Geometry check sheet. Reference: the model listing, model coordinates, mm. Face numbers are marked on the shaded views. A direction names the side the tool comes from. Round coordinates to 2 decimals unless told otherwise and drop trailing zeros. Order: outer loops, then holes, each group sorted by start corner. A loop starts at its lowest first (then second) coordinate and runs counter-clockwise, first axis right, second up.
(1) Cross-section at B-B on x = -2.5. Enter the section's corners in (y, z), and give its area (3 significant figures).
(2) Cross-section at C-C on x = 3.5. Enter the section's corners in (y, z), and give its area (4 significant figures).
(3) Gauge pin test, flat ends, axial feed: P1, Ø3, axis at x = -2.5, z = 4, coming from the -Y side; P2, Ø2, axis at x = -2.5, z = 4, coming from the -Y side. Record the tip position at first contact, or that the pin passes through.
(4) Cross-section at A-A on y = -4.25. Enter the section's corners in (x, z), and give its area (3 significant figures).
(5) Thickness scan on L1, parallel to X at y = -6, z = 4; L2, parallel to X at y = 4.25, z = 1.75; L3, parallel to Y at x = -2.75, z = 5. Record the ranges inside material, lowest first.
(6) Cross-section at D-D on z = 4.5. Enter the section's corners in (x, y).
(7) Draft check along X on the marked faces 1, 2 and 3. Enter one of: pulls with the +X half, pulls with the -X half, needs draft (parallel to the pull), parting line crosses it, or undercut.
(8) Set-up check for the marked faces 4 and 5: record each of +Z, -Z, +X, -X, +Y, -Y from which the full face is reachable in a straight line by a thin tool's end or side.
from build123d import *

# Parameters (mm, degrees)
SKETCH_1_W          = 12.7
SKETCH_1_H          = 15
EXTRUDE_1_DEPTH     = 8
SKETCH_2_R          = 0.75
CUT_EXTRUDE_1_DEPTH = 8
SKETCH_3_R          = 1.25
CUT_EXTRUDE_2_DEPTH = 5


with BuildPart() as part:
    # Эскиз1 → Бобышка-Вытянуть1 (new body)
    with BuildSketch(Plane.XY):
        Rectangle(SKETCH_1_W, SKETCH_1_H)
    extrude(amount=EXTRUDE_1_DEPTH)

    # Эскиз2 → Вырез-Вытянуть1 (cut)
    with BuildSketch(Plane.XY.offset(8)):
        with Locations((-2.3876, 3.786)):
            Circle(SKETCH_2_R)
        with Locations((2.3876, 3.79)):
            Circle(SKETCH_2_R)
    extrude(amount=-CUT_EXTRUDE_1_DEPTH, mode=Mode.SUBTRACT)

    # Эскиз3 → Вырез-Вытянуть2 (cut)
    with BuildSketch(Plane.XZ.offset(7.5)):
        with Locations(Location((-2.5, 4, 0), (0, 0, 270))):
            Circle(SKETCH_3_R)
        with Locations(Location((2.5, 4, 0), (0, 0, 270))):
            Circle(SKETCH_3_R)
    extrude(amount=-CUT_EXTRUDE_2_DEPTH, mode=Mode.SUBTRACT)


solid = part.part
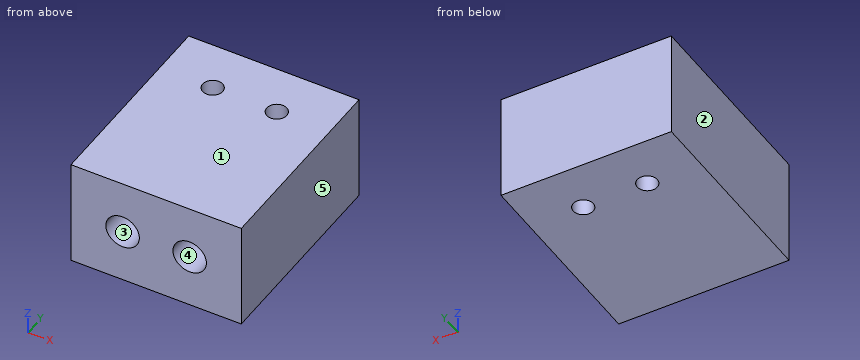
Found:
1. outline: (-7.5, 0) - (3.04, 0) - (3.04, 8) - (-7.5, 8) - (-7.5, 5.25) - (-2.5, 5.25) - (-2.5, 2.75) - (-7.5, 2.75) - close; (4.53, 0) - (7.5, 0) - (7.5, 8) - (4.53, 8) - close
1. area: 95.6 mm2
2. outline: (-7.5, 0) - (7.5, 0) - (7.5, 8) - (-7.5, 8) - (-7.5, 4.75) - (-2.5, 4.75) - (-2.5, 3.25) - (-7.5, 3.25) - close
2. area: 112.5 mm2
3. P1: stops at y = -7.5
3. P2: stops at y = -2.5
4. outline: (-6.35, 0) - (6.35, 0) - (6.35, 8) - (-6.35, 8) - close; hole circle Ø2.5 at (-2.5, 4); hole circle Ø2.5 at (2.5, 4)
4. area: 91.8 mm2
5. L1: x = -6.35 to -3.75, -1.25 to 1.25, 3.75 to 6.35
5. L2: x = -6.35 to -2.98, -1.8 to 1.8, 2.98 to 6.35
5. L3: y = -2.5 to 3.13, 4.44 to 7.5
6. outline: (-6.35, -7.5) - (-3.65, -7.5) - (-3.65, -2.5) - (-1.35, -2.5) - (-1.35, -7.5) - (1.35, -7.5) - (1.35, -2.5) - (3.65, -2.5) - (3.65, -7.5) - (6.35, -7.5) - (6.35, 7.5) - (-6.35, 7.5) - close; hole circle Ø1.5 at (-2.39, 3.79); hole circle Ø1.5 at (2.39, 3.79)
7. face 1: needs draft
7. face 2: pulls with the -X half
7. face 3: undercut
8. face 4: -Y
8. face 5: +Z, -Z, +X, +Y, -Y
